```python
from build123d import *

# Parameters (mm, degrees)
SKETCH1_W             = 73.7
SKETCH1_H             = 73.7
SKETCH1_R             = 3.175
SKETCH1_R_2           = 5
SKETCH1_R_3           = 1.604776926
OPTICAL_MOUNT_DEPTH   = 6.477
F_8_32_TAPPED_HOLE1_D = 3.4544


with BuildPart() as part:
    # Sketch1 → optical_mount (new body)
    with BuildSketch(Plane(origin=(0, 0, 0), x_dir=(1, 0, 0), z_dir=(0, 1, 0))):
        Rectangle(SKETCH1_W, SKETCH1_H)
        with Locations((0, 25.4)):
            Circle(SKETCH1_R, mode=Mode.SUBTRACT)
        with Locations((25.4, 0)):
            Circle(SKETCH1_R, mode=Mode.SUBTRACT)
        with Locations((0, -25.4)):
            Circle(SKETCH1_R, mode=Mode.SUBTRACT)
        with Locations((-25.4, 0)):
            Circle(SKETCH1_R, mode=Mode.SUBTRACT)
        Circle(SKETCH1_R_2, mode=Mode.SUBTRACT)
        with Locations((24.309899871, 33.48518084)):
            Circle(SKETCH1_R_3, mode=Mode.SUBTRACT)
        with Locations((-21.487964718, 33.48518084)):
            Circle(SKETCH1_R_3, mode=Mode.SUBTRACT)
        with Locations((-31.85729255, 24.597185555)):
            Circle(SKETCH1_R_3, mode=Mode.SUBTRACT)
        with Locations((-31.85729255, -23.793010992)):
            Circle(SKETCH1_R_3, mode=Mode.SUBTRACT)
    extrude(amount=OPTICAL_MOUNT_DEPTH)

    # #8-32 Tapped Hole1 (through all)
    with Locations(Plane(origin=(-18.08, 6.477, 0), x_dir=(0, 0, 1), z_dir=(0, 1, 0))):
        with Locations((0, 0), (0, 36.16)):
            Hole(F_8_32_TAPPED_HOLE1_D / 2)


solid = part.part
```
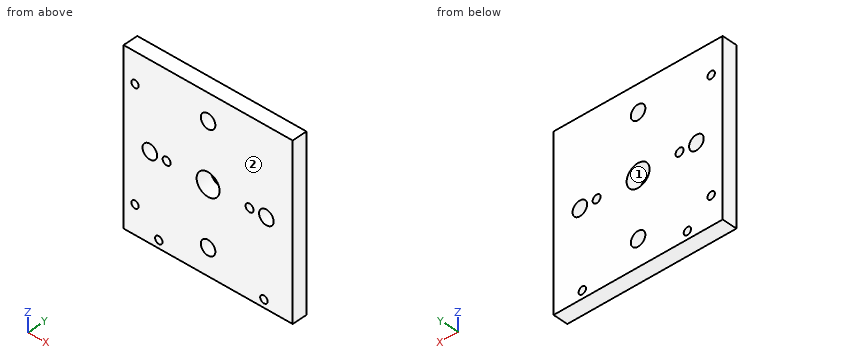
Source: CAD feature listing. Evaluate the final solid. Frame: model axes, mm. Face numbers are marked on the shaded views. Coordinates: 2 decimals unless noted, no trailing zeros. Loops run counter-clockwise (first coordinate to the right, second up) from the corner with the lowest first, then second, coordinate; pieces in that order, holes last. Notation, with made-up numbers: M 34,-27 L 54,-27 A30 cw 54,0 Z; hole C -12,64.25 d11. An arc over 180 degrees is marked long. Use a Markdown table: item, result. Add a question column.
Q1. Material intervals for L1, parallel to X at y = 2, z = 0 (3 decimals); L2, parallel to Z at x = 0, y = 5 (3 decimals); L3, parallel to X at y = 3.5, z = -25.4 (3 decimals), sorted ascending.
Q2. Section query D-D, the plane y = 1.25. State how many separate pieces and enclosed holes the cut face has, and give its area (3 significant figures).
Q3. Section query C-C, the plane x = -1.5. Return loops of the section in (y, z), and give its area (3 significant figures).
Q4. Section query B-B, the plane x = -25.4. Return loops of the section in (y, z) (3 decimals), and give its area (3 significant figures).
Q5. Section query A-A, the plane z = 0. Return loops of the section in (x, y) (3 decimals).
Q6. Draft query along Z for the marked faces 1 and 2. Return one class per face: pulls with the +Z half, pulls with the -Z half, needs draft (parallel to the pull), parting line crosses it, or undercut.
Result:
| question | item | result |
|---|---|---|
| 1 | L1 | x = -36.85 to -28.575, -22.225 to -19.807, -16.353 to -5, 5 to 16.353, 19.807 to 22.225, 28.575 to 36.85 |
| 1 | L2 | z = -36.85 to -28.575, -22.225 to -5, 5 to 22.225, 28.575 to 36.85 |
| 1 | L3 | x = -36.85 to -33.247, -30.468 to -3.175, 3.175 to 36.85 |
| 2 | separate pieces | 1 |
| 2 | enclosed holes | 11 |
| 2 | area | 5,180 mm2 |
| 3 | outline | M 0,-36.85 L 6.48,-36.85 L 6.48,-28.2 L 0,-28.2 Z; M 0,-22.6 L 6.48,-22.6 L 6.48,-4.77 L 0,-4.77 Z; M 0,4.77 L 6.48,4.77 L 6.48,22.6 L 0,22.6 Z; M 0,28.2 L 6.48,28.2 L 6.48,36.85 L 0,36.85 Z |
| 3 | area | 343 mm2 |
| 4 | outline | M 0,-36.85 L 6.477,-36.85 L 6.477,-3.175 L 0,-3.175 Z; M 0,3.175 L 6.477,3.175 L 6.477,36.85 L 0,36.85 Z |
| 4 | area | 436 mm2 |
| 5 | outline | M -36.85,0 L -28.575,0 L -28.575,6.477 L -36.85,6.477 Z; M -22.225,0 L -19.807,0 L -19.807,6.477 L -22.225,6.477 Z; M -16.353,0 L -5,0 L -5,6.477 L -16.353,6.477 Z; M 5,0 L 16.353,0 L 16.353,6.477 L 5,6.477 Z; M 19.807,0 L 22.225,0 L 22.225,6.477 L 19.807,6.477 Z; M 28.575,0 L 36.85,0 L 36.85,6.477 L 28.575,6.477 Z |
| 6 | face 1 | undercut |
| 6 | face 2 | needs draft |
